```python
from build123d import *

# Parameters (mm, degrees)
SALIENTE_EXTRUIR1_DEPTH = 7
CROQUIS3_R              = 4
CORTAR_EXTRUIR1_DEPTH   = 7


with BuildPart() as part:
    # Croquis1 → Saliente-Extruir1 (new body)
    with BuildSketch(Plane.XY):
        Polygon((7.505553499, 0), (3.75277675, 6.5), (-3.75277675, 6.5), (-7.505553499, 0), (-3.75277675, -6.5), (3.75277675, -6.5), align=None)
    extrude(amount=SALIENTE_EXTRUIR1_DEPTH)

    # Croquis2 → Revolución1 (revolve)
    with BuildSketch(Plane(origin=(0, 0, 0), x_dir=(0, 0, -1), z_dir=(1, 0, 0))):
        with BuildLine():
            Line((0, 0), (6, 0))
            ThreePointArc((6, 0), (4.270697462, -4.422951503), (0, -6.5))
            Line((0, -6.5), (0, 0))
        make_face()
    revolve(axis=Axis((0, 0, 0), (0, 0, -1)))

    # Croquis3 → Cortar-Extruir1 (cut)
    with BuildSketch(Plane.XY.offset(7)):
        Circle(CROQUIS3_R)
    extrude(amount=-CORTAR_EXTRUIR1_DEPTH, mode=Mode.SUBTRACT)


solid = part.part
```
Work out the finished part from the listing and answer in its coordinate system (mm). A direction names the side the tool comes from. Give positions to 0.01 mm unless a question says otherwise; leave off trailing zeros. Loops run counter-clockwise (first coordinate to the right, second up) from the corner with the lowest first, then second, coordinate; pieces in that order, holes last. Notation, with made-up numbers: (-26, 56.25) -> (5, 56.25) arc R20 cw to (5, 79.25) -> close; hole circle Ø1 at (37.25, 72.5). An arc over 180 degrees is marked (long way). Put each result on its own line as item: value. Start each with the question number.
Item 1: The part is cut by section C-C (x = 2.5). Give the vertices of the cut face in (y, z), then the cut area to 3 significant figures.
Item 2: The mould has two halves that part along X. Classify faces 1 (the face through (-5.6, 3.3, 3.5)), 2 (the face through (0, 0, 0)), 3 (the face through (-3, -6, 0)): released by +X, released by -X, zero draft, split by the parting line, or undercut.
Item 3: The part is cut by section D-D (z = -0.5). Give the vertices of the cut face in (x, y).
Item 4: The part is cut by section A-A (z = 4.25). Give the vertices of the cut face in (x, y), then the cut area to 3 significant figures.
Item 5: Each of these flat-tipped pins is pushed along its axis until it touches: P1, Ø2.5, axis at x = -2, y = 1.5, coming from the +Z side; P2, Ø2, axis at y = 0.5, z = -3.5, coming from the +X side; P3, Ø3.5, axis at x = 3, y = 4, coming from the -Z side. Where does it stop, or does it pass through?
Item 6: The part is cut by section B-B (y = 0.75). Give the vertices of the cut face in (x, z), then the cut area to 3 significant figures.
Item 7: Find the intervals of material crossed by L1, parallel to Y at x = 0, z = 5.5; L2, parallel to X at y = -3.5, z = 3; L3, parallel to X at y = 3, z = 2.25, in increasing order. Write a range as [from, to].
Item 8: Which of the six approach directions +Z, -Z, +X, -X, +Y, -Y give full straight-line access (tool end or side, diameter ignored) to faces 4 (the face through (7, 0, 0)), 5 (the face through (3, -6, 0)), 6 (the face through (3, 6, 0)), 7 (the face through (-0.867, -3.905, 3.549)), 8 (the face through (-3, 6, 0))?
Answers below:
1. outline: (-6.5, 0) -> (-6, 0) arc R6.02 ccw to (6, 0) -> (6.5, 0) -> (6.5, 7) -> (3.12, 7) -> (3.12, 0) -> (-3.12, 0) -> (-3.12, 7) -> (-6.5, 7) -> close
1. area: 98.0 mm2
2. face 1: released by -X
2. face 2: undercut
2. face 3: zero draft
3. outline: circle Ø12.88 at (0, 0)
4. outline: (-7.51, 0) -> (-3.75, -6.5) -> (3.75, -6.5) -> (7.51, 0) -> (3.75, 6.5) -> (-3.75, 6.5) -> close; hole circle Ø8 at (0, 0)
4. area: 96.1 mm2
5. P1: z = 0
5. P2: x = 5.76
5. P3: z = -5.13
6. outline: (-7.07, 0) -> (-6.46, 0) arc R6.48 ccw to (6.46, 0) -> (7.07, 0) -> (7.07, 7) -> (3.93, 7) -> (3.93, 0) -> (-3.93, 0) -> (-3.93, 7) -> (-7.07, 7) -> close
6. area: 103 mm2
7. L1: [-6.5, -4], [4, 6.5]
7. L2: [-5.48, -1.94], [1.94, 5.48]
7. L3: [-5.77, -2.65], [2.65, 5.77]
8. face 4: -Z, +X
8. face 5: -Z, +X, -Y
8. face 6: -Z, +X, +Y
8. face 7: +Z
8. face 8: -Z, -X, +Y
